Part model, mm, in its own coordinate system. A direction names the side the tool comes from. Coordinates: 2 decimals unless noted, no trailing zeros. Order: outer loops, then holes, each group sorted by start corner. A loop starts at its lowest first (then second) coordinate and runs counter-clockwise, first axis right, second up.
1) Wall check: L1, parallel to Z at x = 190, y = 122; L2, parallel to X at y = 86, z = 425.5; L3, parallel to Z at x = 286.5, y = 94.5. Give the ranges that are in metal, low to high.
2) Mould opens along Z. For faces 1 (the flat face through (188, 203.2, 301)), 2 (the flat face through (188, 177.8, 421)), 3 (the flat face through (188, 103, 0)) say: +Z half, -Z half, draft (parallel to the pull), parting line (faces both ways), or undercut.
3) Cut at D-D (x = 115.5). List the corners of the cut face in (y, z), and give its area (3 significant figures).
4) Cut at B-B (y = 81). List the corners of the cut face in (x, z), and give its area (3 significant figures).
5) Cut at A-A (x = 190.5). List the corners of the cut face in (y, z).
6) Tool access for faces 4 (the flat face through (381, 100, 301)), 5 (the cylindrical face through (154.71, 87.655, 257.926)): list every direction of +Z, -Z, +X, -X, +Y, -Y with a clear straight run to the whole face (end or side of a thin tool).
7) Cut at C-C (z = 461). List the corners of the cut face in (x, y).
```python
from build123d import *

# Parameters (mm, degrees)
F0_W     = 381
F0_H     = 203.2
F1_DEPTH = 609.6
F2_R     = 165.1
F3_DEPTH = 177.8
F4_SIZE  = 5.08


with BuildPart() as f1:
    # F0 (on Top) → F1 (new body)
    with BuildSketch(Plane.XY):
        with Locations((190.5, 101.6)):
            Rectangle(F0_W, F0_H)
    extrude(amount=F1_DEPTH)

    # F2 (on face) → F3 (cut)
    with BuildSketch(Plane.XZ):
        with Locations((190.5, 419.1)):
            Circle(F2_R)
    extrude(amount=-F3_DEPTH, mode=Mode.SUBTRACT)

    # F4
    f4_edges = [f1.edges().sort_by_distance(p)[0] for p in [
        (0, 203.2, 304.8),
        (0, 0, 304.8),
        (381, 0, 304.8),
        (381, 203.2, 304.8),
    ]]
    chamfer(f4_edges, length=F4_SIZE)


solid = f1.part
```
Geometry check:
1. L1: z = 0 to 254, 584.2 to 609.6
1. L2: x = 0 to 25.52, 355.48 to 381
1. L3: z = 0 to 284.78, 553.42 to 609.6
2. face 1: draft
2. face 2: undercut
2. face 3: -Z half
3. outline: (0, 0) - (203.2, 0) - (203.2, 609.6) - (0, 609.6) - (0, 566.18) - (177.8, 566.18) - (177.8, 272.02) - (0, 272.02) - close
3. area: 71,600 mm2
4. outline: (0, 0) - (381, 0) - (381, 609.6) - (0, 609.6) - close; hole circle Ø330.2 at (190.5, 419.1)
4. area: 147,000 mm2
5. outline: (0, 0) - (203.2, 0) - (203.2, 609.6) - (0, 609.6) - (0, 584.2) - (177.8, 584.2) - (177.8, 254) - (0, 254) - close
6. face 4: +Z, -Z, +X, +Y, -Y
6. face 5: -Y
7. outline: (0, 5.08) - (5.08, 0) - (30.81, 0) - (30.81, 177.8) - (350.19, 177.8) - (350.19, 0) - (375.92, 0) - (381, 5.08) - (381, 198.12) - (375.92, 203.2) - (5.08, 203.2) - (0, 198.12) - close
